```python
from build123d import *

# Parameters (mm, degrees)
F1_ANGLE  = 120
F2_R      = 1.6
F3_DEPTH  = 5
F6_W      = 12.938
F6_H      = 7.452
F7_DEPTH  = 1
F8_W      = 13.007
F8_H      = 7.97
F9_DEPTH  = 1
F11_DEPTH = 5


with BuildPart() as f1:
    # F0 (on Front) → F1 (revolve)
    with BuildSketch(Plane.XZ):
        Polygon((23, 5), (15.5, 5), (15.5, 6.5), (11, 6.5), (11, 2.3), (13.5, 2.3), (13.5, 0), (23, 0), align=None)
    revolve(axis=Axis((0, 0, 3.7848940119), (0, 0, 1)), revolution_arc=F1_ANGLE)

    # F2 (on face) → F3 (cut, through all)
    with BuildSketch(Plane.XY.offset(5)):
        with Locations((1.743114855, 19.9238939618)):
            Circle(F2_R)
        with Locations((16.3830408858, 11.471528727)):
            Circle(F2_R)
    extrude(amount=-F3_DEPTH, mode=Mode.SUBTRACT)

    # F6 (on offset) → F7 (cut, through all)
    with BuildSketch(Plane.XZ.offset(-1)):
        with Locations((17.1259158669, 3.1437808403)):
            Rectangle(F6_W, F6_H)
    extrude(amount=F7_DEPTH, mode=Mode.SUBTRACT)

    # F8 (on offset) → F9 (cut, through all)
    with BuildSketch(Plane(origin=(0.8660254038, 0.5, 0), x_dir=(0.5, -0.8660254038, 0), z_dir=(-0.8660254038, -0.5, 0))):
        with Locations((-17.1034485545, 3.2673813227)):
            Rectangle(F8_W, F8_H)
    extrude(amount=F9_DEPTH, mode=Mode.SUBTRACT)

    # F10 (on face) → F11 (cut, through all)
    with BuildSketch(Plane.XY.offset(5)):
        with BuildLine():
            Line((18.9782505862, 1), (22.9782505862, 1))
            ThreePointArc((22.9782505862, 1), (22.6876135739, 3.777855254), (22.0624114729, 6.5))
            Line((22.0624114729, 6.5), (18.0624114729, 6.5))
            Line((18.0624114729, 6.5), (18.9782505862, 1))
        make_face()
        with BuildLine():
            ThreePointArc((22.0624114729, 6.5), (22.6876135739, 3.777855254), (22.9782505862, 1))
            Line((22.9782505862, 1), (23.6873179674, 0.9982389165))
            Line((23.6873179674, 0.9982389165), (23.6873179674, 6.5))
            Line((23.6873179674, 6.5), (22.0624114729, 6.5))
        make_face()
    extrude(amount=-F11_DEPTH, mode=Mode.SUBTRACT)


solid = f1.part
```
Work out the finished part from the listing and answer in its coordinate system (mm). A direction names the side the tool comes from. Round coordinates to 2 decimals unless told otherwise and drop trailing zeros. Order: outer loops, then holes, each group sorted by start corner. A loop starts at its lowest first (then second) coordinate and runs counter-clockwise, first axis right, second up.
Q1. A cutting plane is placed at B-B, the plane z = 1.5. Determine the outline of the cut face in (x, y), then the cut area to 3 significant figures.
Solution:
outline: (-10.62, 20.4) - (-5.87, 12.16) arc R13.5 cw to (13.46, 1) - (18.98, 1) - (18.06, 6.5) - (22.06, 6.5) arc R23 ccw to start; hole circle Ø3.2 at (1.74, 19.92); hole circle Ø3.2 at (16.38, 11.47)
area: 305 mm2
Q2. The mould has two halves that part along Y. Classify faces 1 (the cylindrical face through (7.93, 13.32, 5.76)), 2 (the flat face through (6, 15, 0)), 3 (the cylindrical face through (5.63, 9.45, 4.37)), 4 (the flat face through (20, 6.5, 3)): pulls with the +Y half, pulls with the -Y half, needs draft (parallel to the pull), parting line crosses it, or undercut.
Solution:
face 1: pulls with the +Y half
face 2: needs draft
face 3: pulls with the -Y half
face 4: undercut
Q3. Given pin 1 Ø2 at (y, z) = (4.5, 5) entering from +X, flat-ended and moving along its own axis, determine where the tip first touches the part or whether it passes through.
Solution:
pin 1: stops at x = 18.56
Q4. A cutting plane is placed at C-C, the plane x = 4. Determine the outline of the cut face in (y, z).
Solution:
outline: (10.25, 2.3) - (12.89, 2.3) - (12.89, 0) - (22.65, 0) - (22.65, 5) - (14.97, 5) - (14.97, 6.5) - (10.25, 6.5) - close
Q5. A tool of negligible diameter and unlimited length cuts with its end or side. For faces 5 (the flat face through (-7.66, 15.27, 3.3)), 6 (the flat face through (18.514, 3.788, 2.535)), 7 (the cylindrical face through (6.909, 11.598, 1.134)), from which of +Z, -Z, +X, -X, +Y, -Y can it reach the whole face along a straight path? Write none if from no direction.
Solution:
face 5: +Z, -Z, -X, -Y
face 6: +Z, -Z, +X
face 7: -Z, -Y
Q6. A cutting plane is placed at A-A, the plane y = 19.25. Determine the outline of the cut face in (x, z), then the cut area to 3 significant figures.
Solution:
outline: (-9.96, 0) - (0.29, 0) - (0.29, 5) - (-9.96, 5) - close; (3.19, 0) - (12.59, 0) - (12.59, 5) - (3.19, 5) - close
area: 98.2 mm2
Q7. Find the intervals of material crossed by line 1 along X through (y, z) = (12.25, 1.5); line 2 along Z through (x, y) = (9.5, 6.75); line 3 along X through (y, z) = (19, 1.5), in increasing order.
Solution:
line 1: x = -5.92 to -5.67, 5.67 to 14.99, 17.78 to 19.47
line 2: z = 2.3 to 6.5
line 3: x = -9.81 to 0.44, 3.05 to 12.96
Q8. A cutting plane is placed at D-D, the plane y = 9.25. Determine the outline of the cut face in (x, z).
Solution:
outline: (5.95, 2.3) - (9.83, 2.3) - (9.83, 0) - (21.06, 0) - (21.06, 5) - (12.44, 5) - (12.44, 6.5) - (5.95, 6.5) - close
